```python
from build123d import *

# Parameters (mm, degrees)
PAD_DEPTH       = 12
SKETCH001_R     = 2.6
POCKET_DEPTH    = 4
SKETCH002_R     = 1.6
POCKET001_DEPTH = 10
FILLET_R        = 1
SKETCH003_W     = 8
SKETCH003_H     = 5.2
POCKET002_DEPTH = 5


with BuildPart() as part:
    # Sketch → Pad (new body)
    with BuildSketch(Plane.XY):
        Polygon((-4, 9.1), (10, 9.1), (10, 6.1), (0, 6.1), (0, 3), (10, 3), (10, 0), (0, 0), (0, -2.971797), (4, -9.9), (16, -9.9), (16, -13.9), (1.690599, -13.9), (-4, -4.043594), align=None)
    extrude(amount=PAD_DEPTH)

    # Sketch001 (on Face13 of Pad) → Pocket (cut)
    with BuildSketch(Plane.XZ.offset(13.9)):
        with Locations((10, 6)):
            Circle(SKETCH001_R)
    extrude(amount=-POCKET_DEPTH, mode=Mode.SUBTRACT)

    # Sketch002 (on Face2 of Pocket) → Pocket001 (cut)
    with BuildSketch(Plane(origin=(0, 9.1, 0), x_dir=(-1, 0, 0), z_dir=(0, 1, 0))):
        with Locations((-5, 6)):
            Circle(SKETCH002_R)
    extrude(amount=-POCKET001_DEPTH, mode=Mode.SUBTRACT)

    # Fillet
    fillet_edges = [part.edges().sort_by_distance(p)[0] for p in [
        (10, 1.5, 12),
        (10, 7.6, 12),
        (10, 7.6, 0),
        (10, 1.5, 0),
        (16, -11.9, 12),
        (16, -11.9, 0),
    ]]
    fillet(fillet_edges, radius=FILLET_R)

    # Sketch003 (on Face16 of Fillet) → Pocket002 (cut)
    with BuildSketch(Plane(origin=(0, -9.9, 0), x_dir=(-1, 0, 0), z_dir=(0, 1, 0))):
        with Locations((-14, 6)):
            Rectangle(SKETCH003_W, SKETCH003_H)
    extrude(amount=-POCKET002_DEPTH, mode=Mode.SUBTRACT)


solid = part.part
```
Design review of the part built by this model. Coordinates are the model's own, in mm. A direction names the side the tool comes from. Coordinates: 2 decimals unless noted, no trailing zeros. Order: outer loops, then holes, each group sorted by start corner. A loop starts at its lowest first (then second) coordinate and runs counter-clockwise, first axis right, second up. Notation, with made-up numbers: (5.25, 64) - (64.25, 64) arc R15 cw to (64.25, 81) - close; hole circle Ø1 at (-11, 76.25). An arc over 180 degrees is marked (long way). One line per question, with ' | ' between items.
Q1. Consider section A-A, the plane z = 6. Give the boundary of the cut face in (x, y).
Answer key:
outline: (-4, -4.04) - (1.69, -13.9) - (7.4, -13.9) - (7.4, -9.9) - (4, -9.9) - (0, -2.97) - (0, 0) - (3.4, 0) - (3.4, 3) - (0, 3) - (0, 6.1) - (3.4, 6.1) - (3.4, 9.1) - (-4, 9.1) - close; (6.6, 0) - (10, 0) - (10, 3) - (6.6, 3) - close; (6.6, 6.1) - (10, 6.1) - (10, 9.1) - (6.6, 9.1) - close
Q2. Clearance check with flat-ended pins moving along their axes: pin 1 Ø2.5 at (y, z) = (7.5, 6) entering from +X; pin 2 Ø4 at (x, z) = (5, 6) entering from +Y; pin 3 Ø5 at (x, z) = (-1, 7.5) entering from -Y; pin 4 Ø2.5 at (x, z) = (5, 6) entering from +Y. State where each tip first meets the part, or that it passes through.
Answer key:
pin 1: stops at x = 10 | pin 2: stops at y = 9.1 | pin 3: stops at y = -13.57 | pin 4: stops at y = -9.47
Q3. Consider section B-B, the plane x = 5. Give the boundary of the cut face in (y, z), then the cut area to 3 significant figures.
Answer key:
outline: (-13.9, 0) - (-9.9, 0) - (-9.9, 12) - (-13.9, 12) - close; (0, 0) - (3, 0) - (3, 4.4) - (0, 4.4) - close; (0, 7.6) - (3, 7.6) - (3, 12) - (0, 12) - close; (6.1, 0) - (9.1, 0) - (9.1, 4.4) - (6.1, 4.4) - close; (6.1, 7.6) - (9.1, 7.6) - (9.1, 12) - (6.1, 12) - close | area: 101 mm2
Q4. To check wall thickness, follow line 1 along Y through (x, z) = (6.25, 3.75); line 2 along Y through (x, z) = (1, 1); line 3 along Z through (x, y) = (5, 1.8). State the ranges of each line that lie inside material, in increasing order.
Answer key:
line 1: y = -13.9 to -9.9, 0 to 3, 6.1 to 9.1 | line 2: y = -12.7 to -4.7, 0 to 3, 6.1 to 9.1 | line 3: z = 0 to 4.4, 7.6 to 12
Q5. Consider section C-C, the plane x = 9.5. Give the boundary of the cut face in (y, z), then the cut area to 3 significant figures.
Answer key:
outline: (-13.9, 0) - (-9.9, 0) - (-9.9, 3.45) - (-13.9, 3.45) - close; (-13.9, 8.55) - (-9.9, 8.55) - (-9.9, 12) - (-13.9, 12) - close; (0, 0.13) - (3, 0.13) - (3, 11.87) - (0, 11.87) - close; (6.1, 0.13) - (9.1, 0.13) - (9.1, 11.87) - (6.1, 11.87) - close | area: 98.0 mm2
Q6. For faces 4 (the cylindrical face through (7.4, -11.9, 6.1)), 5 (the cylindrical face through (6.27, 7.62, 5.03)), 6 (the cylindrical face through (9.699, 7.579, 0.285)), 7 (the flat face through (13, -12, 3.4)), 8 (the flat face through (6.2, 6.1, 4.6)), list the 3-axis set-ups (+Z, -Z, +X, -X, +Y, -Y) from which the entire face can be reached by the end or side of a thin tool; tool diameter is ignored.
Answer key:
face 4: +X, -Y | face 5: +Y | face 6: -Z, +X, +Y | face 7: +X, +Y, -Y | face 8: +Z, -Z, +X
Q7. The part is to be moulded in two halves that separate along Y. For faces 1 (the flat face through (7, -13.9, 6)), 2 (the flat face through (13, -12, 8.6)), 3 (the flat face through (1.972, -6.387, 5.916)), say which applies: +Y half, -Y half, draft (parallel to the pull), parting line (faces both ways), or undercut.
Answer key:
face 1: -Y half | face 2: draft | face 3: undercut
Q8. Consider section D-D, the plane z = 1.5. Give the boundary of the cut face in (x, y).
Answer key:
outline: (-4, -4.04) - (1.69, -13.9) - (16, -13.9) - (16, -9.9) - (4, -9.9) - (0, -2.97) - (0, 0) - (10, 0) - (10, 3) - (0, 3) - (0, 6.1) - (10, 6.1) - (10, 9.1) - (-4, 9.1) - close
